from build123d import *

# Parameters (mm, degrees)
F0_R     = 11.05
F1_DEPTH = 7


# Not quite as in the source:
# - a feature names something its author has since deleted; it is built from what else it names


with BuildPart() as f1:
    # F0 (on Top) → F1 (new body)
    with BuildSketch(Plane.XY):
        with BuildLine():
            ThreePointArc((-19.2783924252, 3.2977389637), (-20.321649546, -2.3852041509), (-23.3153727308, -7.3270509067))
            ThreePointArc((-23.3153727308, -7.3270509067), (-15.247882117, -8.2153155431), (-8.1783924252, -12.2022610363))
            ThreePointArc((-8.1783924252, -12.2022610363), (-1.221278488, -8.1070481694), (6.7932734583, -7.1379455637))
            ThreePointArc((6.7932734583, -7.1379455637), (2.9292273158, 3.7914733565), (7.4601219716, 14.4617144101))
            ThreePointArc((7.4601219716, 14.4617144101), (1.8212672524, 15.0889872554), (-1.9835406039, 19.2977389637))
            Line((-1.9835406039, 19.2977389637), (-14.3732442464, 19.2977389637))
            ThreePointArc((-14.3732442464, 19.2977389637), (-18.1780521028, 15.0889872554), (-23.816906822, 14.4617144101))
            ThreePointArc((-23.816906822, 14.4617144101), (-20.4563856506, 9.3233605229), (-19.2783924252, 3.2977389637))
        make_face()
        with Locations((-8.1783924252, 3.2977389637)):
            Circle(F0_R, mode=Mode.SUBTRACT)
        with BuildLine():
            ThreePointArc((-28.490516072, 17.7865185747), (-31.8013587595, 18.915364804), (-35.2783924252, 19.2977389637))
            ThreePointArc((-35.2783924252, 19.2977389637), (-51.2783924252, 3.2977389637), (-35.2783924252, -12.7022610363))
            ThreePointArc((-35.2783924252, -12.7022610363), (-29.74444778, -9.0185588521), (-23.3153727308, -7.3270509067))
            ThreePointArc((-23.3153727308, -7.3270509067), (-20.321649546, -2.3852041509), (-19.2783924252, 3.2977389637))
            ThreePointArc((-19.2783924252, 3.2977389637), (-20.4563856506, 9.3233605229), (-23.816906822, 14.4617144101))
            ThreePointArc((-23.816906822, 14.4617144101), (-26.4619172405, 15.6908779087), (-28.490516072, 17.7865185747))
        make_face()
        with Locations((-35.2783924252, 3.2977389637)):
            Circle(F0_R, mode=Mode.SUBTRACT)
        with BuildLine():
            ThreePointArc((7.4601219716, 14.4617144101), (2.9292273158, 3.7914733565), (6.7932734583, -7.1379455637))
            ThreePointArc((6.7932734583, -7.1379455637), (13.3416443494, -8.8647019853), (18.9216075748, -12.7022610363))
            ThreePointArc((18.9216075748, -12.7022610363), (30.2353160738, -8.0159695352), (34.9216075748, 3.2977389637))
            ThreePointArc((34.9216075748, 3.2977389637), (30.2353160738, 14.6114474627), (18.9216075748, 19.2977389637))
            ThreePointArc((18.9216075748, 19.2977389637), (15.4445739091, 18.915364804), (12.1337312216, 17.7865185747))
            ThreePointArc((12.1337312216, 17.7865185747), (10.1051323901, 15.6908779087), (7.4601219716, 14.4617144101))
        make_face()
        with Locations((18.9216075748, 3.2977389637)):
            Circle(F0_R, mode=Mode.SUBTRACT)
        with BuildLine():
            Line((-29.2757110635, 19.2977389637), (-35.2783924252, 19.2977389637))
            ThreePointArc((-35.2783924252, 19.2977389637), (-31.8013587595, 18.915364804), (-28.490516072, 17.7865185747))
            ThreePointArc((-28.490516072, 17.7865185747), (-28.923441503, 18.5211753113), (-29.2757110635, 19.2977389637))
        make_face()
        with BuildLine():
            Line((18.9216075748, 19.2977389637), (12.9189262131, 19.2977389637))
            ThreePointArc((12.9189262131, 19.2977389637), (12.5666566526, 18.5211753113), (12.1337312216, 17.7865185747))
            ThreePointArc((12.1337312216, 17.7865185747), (15.4445739091, 18.915364804), (18.9216075748, 19.2977389637))
        make_face()
        with BuildLine():
            ThreePointArc((-13.824477655, 22.2096319377), (-13.9628662658, 20.7280563015), (-14.3732442464, 19.2977389637))
            Line((-14.3732442464, 19.2977389637), (-1.9835406039, 19.2977389637))
            ThreePointArc((-1.9835406039, 19.2977389637), (-2.5323071954, 22.2096319377), (-1.9835406039, 25.1215249117))
            Line((-1.9835406039, 25.1215249117), (-3.9835406039, 23.4114221363))
            ThreePointArc((-3.9835406039, 23.4114221363), (-8.1817639697, 21.709585029), (-12.3732442464, 23.4279627693))
            Line((-12.3732442464, 23.4279627693), (-14.0983548132, 25.1215249117))
            Line((-14.0983548132, 25.1215249117), (-14.3732442464, 25.1215249117))
            ThreePointArc((-14.3732442464, 25.1215249117), (-13.9628662658, 23.691207574), (-13.824477655, 22.2096319377))
        make_face()
    extrude(amount=F1_DEPTH)


solid = f1.part
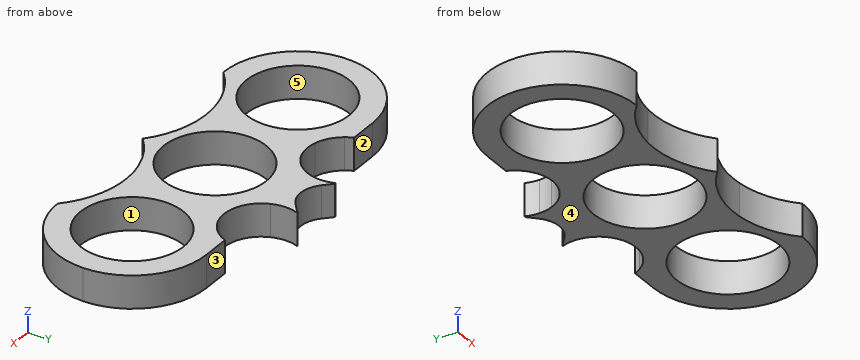
Work out the finished part from the listing and answer in its coordinate system (mm). Face numbers are marked on the shaded views. A direction names the side the tool comes from. Give positions to 0.01 mm unless a question says otherwise; leave off trailing zeros. Loops run counter-clockwise (first coordinate to the right, second up) from the corner with the lowest first, then second, coordinate; pieces in that order, holes last. Notation, with made-up numbers: M 49.25,-36 L 54.25,-36 A9 cw 54.25,-30 Z; hole C -12.75,75 d6. An arc over 180 degrees is marked long. Use CSV: the item, a comma, the result in double quotes.
1) Find section A-A on z = 3.75. Write down the section's boundary in (x, y).
Answer:
outline,"M -35.28,-12.7 A20.23 cw -8.18,-12.2 A19.75 cw 18.92,-12.7 A16 ccw 18.92,19.3 L 12.92,19.3 A8 cw -1.98,25.12 L -3.98,23.41 A6 cw -12.37,23.43 L -14.1,25.12 L -14.37,25.12 A8 cw -29.28,19.3 L -35.28,19.3 A16 ccw Z; hole C -35.28,3.3 d22.1; hole C -8.18,3.3 d22.1; hole C 18.92,3.3 d22.1"
2) Given P1, Ø4, axis at x = -11.5, z = 2, coming from the +Y side, flat-ended and moving along its own axis, determine where the tip first touches the part or whether it passes through.
Answer:
P1,"y = 24.53"
3) Determine the mould class of the marked faces 3, 4 and 5 for opening direction Y: released by +Y, released by -Y, zero draft, split by the parting line, or undercut.
Answer:
face 3,"released by +Y"
face 4,"zero draft"
face 5,"undercut"
4) Find section D-D on y = -10. Write down the section's boundary in (x, z), plus the area to 3 significant figures.
Answer:
outline,"M -44.18,0 L -31.65,0 L -31.65,7 L -44.18,7 Z; M -11.25,0 L -5.25,0 L -5.25,7 L -11.25,7 Z; M 15.46,0 L 27.82,0 L 27.82,7 L 15.46,7 Z"
area,"216 mm^2"
5) Which of the six approach directions +Z, -Z, +X, -X, +Y, -Y give full straight-line access (tool end or side, diameter ignored) to the marked faces 1 and 2?
Answer:
face 1,"+Z, -Z"
face 2,"+Z, -Z, -X, +Y"
6) Find section C-C on y = 13. Write down the section's boundary in (x, z).
Answer:
outline,"M -48,0 L -40.57,0 L -40.57,7 L -48,7 Z; M -29.99,0 L -13.47,0 L -13.47,7 L -29.99,7 Z; M -2.89,0 L 13.63,0 L 13.63,7 L -2.89,7 Z; M 24.21,0 L 31.64,0 L 31.64,7 L 24.21,7 Z"
7) Consider L1, parallel to X at y = -4, z = 5.5; L2, parallel to X at y = -11, z = 6.25; L3, parallel to Y at x = -35.5, z = 2.5. Determine where each line is inside the solid, lowest interval first.
Answer:
L1,"-49.52 to -43.58, -26.98 to -16.48, 0.12 to 10.62, 27.22 to 33.16"
L2,"-42.46 to -33.2, -9.7 to -6.72, 16.94 to 26.1"
L3,"-12.7 to -7.75, 14.35 to 19.3"
8) Find section B-B on x = 28. Write down the section's boundary in (y, z), plus the area to 3 significant figures.
Answer:
outline,"M -9.88,0 L -3,0 L -3,7 L -9.88,7 Z; M 9.6,0 L 16.47,0 L 16.47,7 L 9.6,7 Z"
area,"96.3 mm^2"
